The model under review builds one solid part; all positions refer to its coordinate system, in mm. Face numbers are marked on the shaded views. A direction names the side the tool comes from. Coordinates: 2 decimals unless noted, no trailing zeros. Write each loop counter-clockwise with the first axis right and the second up, starting at its lowest first coordinate (ties: lowest second). Pieces come first, ordered by that corner, then holes. Notation, with made-up numbers: (-5.5, 47) - (5.5, 47) arc R26 ccw to (5.5, 75) - close; hole circle Ø5 at (-36.75, 0.5). An arc over 180 degrees is marked (long way). Return JSON: item names as keys, results as strings. Group by question number.
(1) We need section B-B on z = 32.5. State the section outline as (x, y) points, then the cut area to 3 significant figures.
(2) Tool access review of the marked faces 4, 5 and 6: name each direction out of +Z, -Z, +X, -X, +Y, -Y from which nothing blocks a thin tool from reaching the whole face with its end or side.
(3) We need section A-A on x = -28. State the section outline as (y, z) points, then the cut area to 3 significant figures.
(4) To check wall thickness, follow L1, parallel to X at y = 4.5, z = 9.5; L2, parallel to Z at x = -28, y = 5; L3, parallel to X at y = -58, z = 3.5. State the ranges of each line that lie inside material, in increasing order. Write a range as from..to.
(5) We need section D-D on x = 0. State the section outline as (y, z) points.
(6) Draft analysis for pull direction Y (two halves, no side actions). For the marked faces 1, 2 and 3, state which applies: released by +Y, released by -Y, zero draft, split by the parting line, or undercut.
(7) For pin 1 Ø6.5 at (x, z) = (28, 9.5) entering from -Y; pin 2 Ø7 at (x, y) = (2.5, 1) entering from +Z; pin 3 Ø12 at (x, z) = (-2, 14.5) entering from -Y; pin 4 Ø8 at (y, z) = (-89, 14.5) entering from -X, all flat-tipped, find the tip position at first contact; note any pin that passes through.
(8) We need section C-C on y = 0. State the section outline as (x, z) points, then the cut area to 3 significant figures.
Autodesk Inventor part; units mm, degrees
ref_plane "YZ Plane" through (0, 0, 0) normal (1, 0, 0) x (0, 1, 0)
ref_plane "XZ Plane" through (0, 0, 0) normal (0, 1, 0) x (-1, 0, 0)
ref_plane "XY Plane" through (0, 0, 0) normal (0, 0, 1) x (1, 0, 0)
sketch "Sketch2" plane through (0, 0, 0) normal (0, 0, 1) x (1, 0, 0)
  line L0 (-40, 16) -> (40, 16)
  line L1 (40, 16) -> (40, -16)
  line L2 (40, -16) -> (-40, -16)
  line L3 (-40, -16) -> (-40, 16)
  line L4 (-40, 16) -> (40, -16) construction
  line L5 (40, 16) -> (-40, -16) construction
  point P0 (0, 0)
  dimension "d4" = 32
  dimension "d5" = 80
extrude "Extrusion1" add sketch "Sketch2" along normal blind 26
sketch "Sketch3" plane through (0, 0, 26) normal (0, 0, 1) x (1, 0, 0)
  circle A0 centre (0, 0) radius 7
  dimension "d8" = 14
extrude "Extrusion2" add sketch "Sketch3" along normal blind 3
sketch "Sketch4" plane through (0, 0, 29) normal (0, 0, 1) x (1, 0, 0)
  circle A0 centre (0, 0) radius 4.95
  dimension "d11" = 9.9
extrude "Extrusion3" add sketch "Sketch4" along normal blind 9
sketch "Sketch6" plane through (-40, 16, 0) normal (0, 1, 0) x (1, 0, 0)
  line L0 (12, -9.5) -> (0, -9.5) construction
  line L1 (0, 0) -> (0, -26)
  line L2 (68, -9.5) -> (80, -9.5) construction
  line L3 (80, 0) -> (80, -26)
  line L4 (80, 0) -> (0, 0)
  point P0 (40, 0)
  point P1 (74, -9.5)
  dimension "d29" = 56
  dimension "d30" = 9.5
hole "Hole3" at (-28, 16, 9.5) at (28, 16, 9.5) direction (0, -1, 0) diameter 8.2 end through all
sketch "Sketch7" plane through (-40, -16, 0) normal (0, -1, 0) x (1, 0, 0)
  line L0 (80, 0) -> (80, 26)
  line L1 (0, 0) -> (0, 26)
  line L2 (80, 0) -> (0, 26)
  point P0 (40, 0)
sketch "Sketch9" plane through (40, -16, 0) normal (1, 0, 0) x (0, 0, -1)
  line L0 (0, 0) -> (0, 32)
  line L1 (0, 32) -> (-26, 32)
  line L2 (-26, 32) -> (-26, -168)
  line L3 (-26, -168) -> (0, -168)
  line L4 (0, -168) -> (0, 32)
  line L5 (-26, 0) -> (-26, 32)
  point P0 (0, 16)
  dimension "d38" = 200
extrude "Extrusion4" add sketch "Sketch9" along normal blind 32
sketch "Sketch11" plane through (40, -184, 0) normal (0, -1, 0) x (1, 0, 0)
  line L0 (32, 0) -> (-30, 0)
  line L1 (32, 62) -> (-30, 0)
  line L2 (32, 0) -> (32, 62)
  point P0 (-40, 0)
  point P1 (0, 0)
  dimension "d43" = 62
  dimension "d44" = 62
extrude "Extrusion5" add sketch "Sketch11" against normal blind 10
fillet "Fillet1" radius 5 2 edges at (10, -179, 0) (72, -179, 62)
sketch "Sketch12" plane through (72, -184, 0) normal (0, -1, 0) x (1, 0, 0)
  line L0 (0, 0) -> (-32, 0)
  line L1 (-32, 0) -> (-32, 32)
  line L2 (-32, 32) -> (0, 32)
  line L3 (0, 32) -> (0, 0)
  circle A0 centre (-44, 9.5) radius 4.1
  line L4 (-49.9289, 0) -> (0, 0)
  line L5 (0, 0) -> (0, 49.9289)
  point P0 (-72, 0)
  point P1 (-8, 42)
  point P2 (-42, 8)
  dimension "d48" = 32
  dimension "d49" = 32
  dimension "d50" = 8
  dimension "d51" = 10
  dimension "d52" = 10
  dimension "d53" = 8
hole "Hole4" at (64, -184, 42) at (30, -184, 8) direction (0, 1, 0) diameter 8.2 depth 20
fillet "Fillet2" radius 10 1 edges at (72, 16, 13)
properties part number "13042026-06"
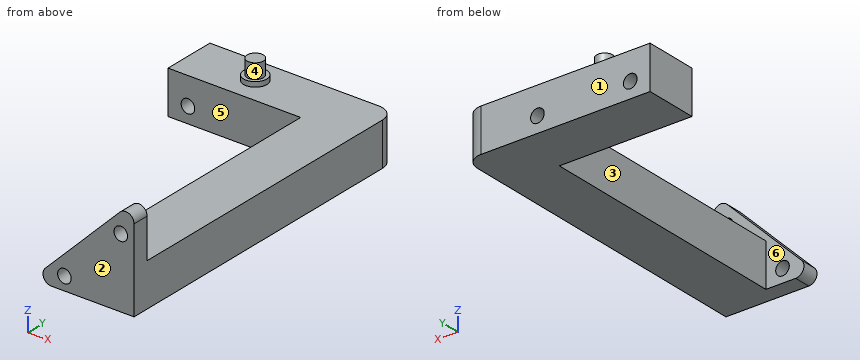
Ans:
{
 "1": {"outline": "circle Ø9.9 at (0, 0); (42.5, -184) - (72, -184) - (72, -174) - (42.5, -174) - close", "area": "372 mm²"},
 "2": {"face 4": "+Z", "face 5": "+Z, -Z, -X", "face 6": "+Z, -X"},
 "3": {"outline": "(-16, 0) - (16, 0) - (16, 5.4) - (-16, 5.4) - close; (-16, 13.6) - (16, 13.6) - (16, 26) - (-16, 26) - close", "area": "570 mm²"},
 "4": {"L1": "-40..-32.1, -23.9..23.9, 32.1..72", "L2": "0..5.4, 13.6..26", "L3": "40..72"},
 "5": {"outline": "(-16, 0) - (16, 0) - (16, 26) - (7, 26) - (7, 29) - (4.95, 29) - (4.95, 38) - (-4.95, 38) - (-4.95, 29) - (-7, 29) - (-7, 26) - (-16, 26) - close"},
 "6": {"face 1": "released by +Y", "face 2": "released by -Y", "face 3": "undercut"},
 "7": {"pin 1": "y = -184", "pin 2": "z = 38", "pin 3": "y = -16", "pin 4": "x = 40"},
 "8": {"outline": "(-40, 0) - (72, 0) - (72, 26) - (7, 26) - (7, 29) - (4.95, 29) - (4.95, 38) - (-4.95, 38) - (-4.95, 29) - (-7, 29) - (-7, 26) - (-40, 26) - close; hole circle Ø8.2 at (-28, 9.5); hole circle Ø8.2 at (28, 9.5)", "area": "2,940 mm²"}
}
